```python
from build123d import *

# Parameters (mm, degrees)
F1_DEPTH = 12.7


# Not quite as in the source:
# - a feature names something its author has since deleted; it is built from what else it names


with BuildPart() as f1:
    # F0 (on Front) → F1 (new body)
    with BuildSketch(Plane.XZ):
        Polygon((5.7657995114, 3.3288859), (0, 6.6577718), (-5.7657995114, 3.3288859), (-5.7657995114, -3.3288859), (0, -6.6577718), (5.7657995114, -3.3288859), align=None)
        with BuildLine():
            ThreePointArc((-1.3748153285, 0.79375), (-0.79375, 1.3748153285), (0, 1.5875))
            ThreePointArc((0, 1.5875), (0.79375, 1.3748153285), (1.3748153285, 0.79375))
            ThreePointArc((1.3748153285, 0.79375), (1.5334072492, 0.4108752341), (1.5875, 0))
            ThreePointArc((1.5875, 0), (1.5334072492, -0.4108752341), (1.3748153285, -0.79375))
            ThreePointArc((1.3748153285, -0.79375), (0.79375, -1.3748153285), (0, -1.5875))
            ThreePointArc((0, -1.5875), (-0.79375, -1.3748153285), (-1.3748153285, -0.79375))
            ThreePointArc((-1.3748153285, -0.79375), (-1.5875, 0), (-1.3748153285, 0.79375))
        make_face(mode=Mode.SUBTRACT)
    extrude(amount=F1_DEPTH)


solid = f1.part
```
Work out the finished part from the listing and answer in its coordinate system (mm). Coordinates: 2 decimals unless noted, no trailing zeros. Write each loop counter-clockwise with the first axis right and the second up, starting at its lowest first coordinate (ties: lowest second). Pieces come first, ordered by that corner, then holes.
Q1. Find the intervals of material crossed by line 1 (X direction, y = -11.25, z = 0.5); line 2 (X direction, y = -7, z = -1.25); line 3 (Z direction, x = 0.75, y = -4.75), in increasing order.
Q2. A cutting plane is placed at B-B, the plane x = -1. Give the vertices of the cut face in (y, z).
Q3. A cutting plane is placed at C-C, the plane z = -1. Give the vertices of the cut face in (x, y).
Q4. A cutting plane is placed at D-D, the plane z = 3.75. Give the vertices of the cut face in (x, y), then the cut area to 3 significant figures.
Q5. This flat-tipped pin is pushed along its axis until it touches: pin 1 Ø5 at (x, y) = (0, -6) entering from -Z. Where does it stop, or does it pass through?
Q6. A cutting plane is placed at A-A, the plane y = -2.5. Give the vertices of the cut face in (x, z) (1 decimal), then the cut area to 3 significant figures.
Findings below:
1. line 1: x = -5.77 to -1.51, 1.51 to 5.77
1. line 2: x = -5.77 to -0.98, 0.98 to 5.77
1. line 3: z = -6.22 to -1.4, 1.4 to 6.22
2. outline: (-12.7, -6.08) - (0, -6.08) - (0, -1.23) - (-12.7, -1.23) - close; (-12.7, 1.23) - (0, 1.23) - (0, 6.08) - (-12.7, 6.08) - close
3. outline: (-5.77, -12.7) - (-1.23, -12.7) - (-1.23, 0) - (-5.77, 0) - close; (1.23, -12.7) - (5.77, -12.7) - (5.77, 0) - (1.23, 0) - close
4. outline: (-5.04, -12.7) - (5.04, -12.7) - (5.04, 0) - (-5.04, 0) - close
4. area: 128 mm2
5. pin 1: stops at z = -6.66
6. outline: (-5.8, -3.3) - (0, -6.7) - (5.8, -3.3) - (5.8, 3.3) - (0, 6.7) - (-5.8, 3.3) - close; hole circle Ø3.2 at (0, 0)
6. area: 107 mm2
